CAD build for the part. Positions are in the model's coordinates, mm. Round coordinates to 2 decimals unless told otherwise and drop trailing zeros. Loops run counter-clockwise (first coordinate to the right, second up) from the corner with the lowest first, then second, coordinate; pieces in that order, holes last. Notation, with made-up numbers: (57.5, 55.5) -> (106.5, 55.5) arc R32 ccw to (106.5, 90.5) -> close; hole circle Ø11 at (-26.75, -40). An arc over 180 degrees is marked (long way). Answer as CSV lines item,"result".
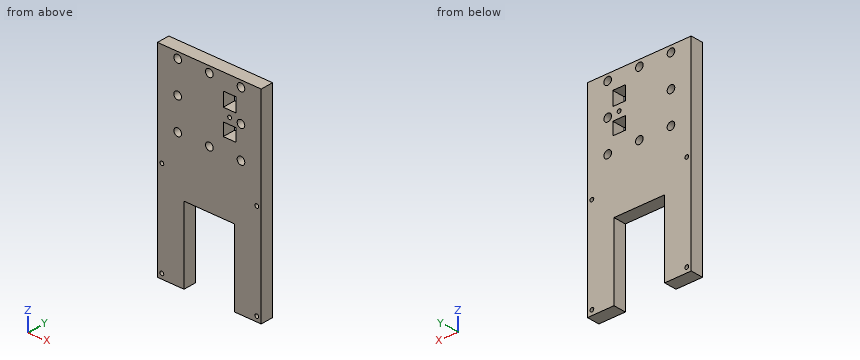
```python
from build123d import *

# Parameters (mm, degrees)
SKETCH1_R           = 3
SKETCH1_R_2         = 1.5
SKETCH1_W           = 10
SKETCH1_H           = 11
SKETCH1_H_2         = 10
BOSS_EXTRUDE1_DEPTH = 10


with BuildPart() as part:
    # Sketch1 → Boss-Extrude1 (new body)
    with BuildSketch(Plane(origin=(0, 0, 0), x_dir=(1, 0, 0), z_dir=(0, 1, 0))):
        Polygon((32.969203123, -64.744115369), (-49.030796877, -64.744115369), (-49.030796877, 95.255884631), (-28.030796877, 95.255884631), (-28.030796877, 35.255884631), (11.969203123, 35.255884631), (11.969203123, 95.255884631), (32.969203123, 95.255884631), align=None)
        with Locations(Location((-33.030796877, -59.744115369, 0), (0, 0, 270))):
            Circle(SKETCH1_R, mode=Mode.SUBTRACT)
        with Locations(Location((16.969203123, -59.744115369, 0), (0, 0, 270))):
            Circle(SKETCH1_R, mode=Mode.SUBTRACT)
        with Locations(Location((16.969203123, -9.744115369, 0), (0, 0, 270))):
            Circle(SKETCH1_R, mode=Mode.SUBTRACT)
        with Locations(Location((-33.030796877, -9.744115369, 0), (0, 0, 270))):
            Circle(SKETCH1_R, mode=Mode.SUBTRACT)
        with Locations(Location((-45.530796877, 91.255884631, 0), (0, 0, 270))):
            Circle(SKETCH1_R_2, mode=Mode.SUBTRACT)
        with Locations(Location((29.469203123, 91.255884631, 0), (0, 0, 270))):
            Circle(SKETCH1_R_2, mode=Mode.SUBTRACT)
        with Locations(Location((29.469203123, 16.255884631, 0), (0, 0, 270))):
            Circle(SKETCH1_R_2, mode=Mode.SUBTRACT)
        with Locations(Location((-45.530796877, 16.255884631, 0), (0, 0, 270))):
            Circle(SKETCH1_R_2, mode=Mode.SUBTRACT)
        with Locations(Location((-8.030796877, -9.744115369, 0), (0, 0, 270))):
            Circle(SKETCH1_R, mode=Mode.SUBTRACT)
        with Locations(Location((-33.030796877, -34.744115369, 0), (0, 0, 270))):
            Circle(SKETCH1_R, mode=Mode.SUBTRACT)
        with Locations(Location((16.969203123, -34.744115369, 0), (0, 0, 270))):
            Circle(SKETCH1_R, mode=Mode.SUBTRACT)
        with Locations(Location((-8.030796877, -59.744115369, 0), (0, 0, 270))):
            Circle(SKETCH1_R, mode=Mode.SUBTRACT)
        with Locations(Location((7.969203123, -35.744115369, 0), (0, 0, 270))):
            Circle(SKETCH1_R_2, mode=Mode.SUBTRACT)
        with Locations((7.969203123, -46.244115369)):
            Rectangle(SKETCH1_W, SKETCH1_H, mode=Mode.SUBTRACT)
        with Locations((7.969203123, -25.744115369)):
            Rectangle(SKETCH1_W, SKETCH1_H_2, mode=Mode.SUBTRACT)
    extrude(amount=BOSS_EXTRUDE1_DEPTH)


solid = part.part
```
Q1. Drop flat-ended pins along their axis: pin 1 Ø2.5 at (x, z) = (29.47, -16.26) entering from -Y; pin 2 Ø5 at (x, y) = (6.5, 3.5) entering from -Z. Give the stop position or say it passes through.
Results:
pin 1,"through"
pin 2,"z = -35.26"
Q2. Slice it at A-A, the plane z = -76. Give the cut face in (x, y), and give its area (3 significant figures).
Results:
outline,"(-49.03, 0) -> (-28.03, 0) -> (-28.03, 10) -> (-49.03, 10) -> close; (11.97, 0) -> (32.97, 0) -> (32.97, 10) -> (11.97, 10) -> close"
area,"420 mm2"
Q3. Probe L1, parallel to Z at x = 17, y = 1; L2, parallel to Z at x = -32.5, y = 4.75; L3, parallel to X at y = 6.5, z = 30.5. List the from-to ranges inside material, lowest first. Write a range as [from, to].
Results:
L1,"[-95.26, 6.74], [12.74, 31.74], [37.74, 56.74], [62.74, 64.74]"
L2,"[-95.26, 6.79], [12.7, 31.79], [37.7, 56.79], [62.7, 64.74]"
L3,"[-49.03, 2.97], [12.97, 32.97]"
Q4. Slice it at C-C, the plane x = -19.5. Give the cut face in (y, z).
Results:
outline,"(0, -35.26) -> (10, -35.26) -> (10, 64.74) -> (0, 64.74) -> close"
Q5. Slice it at B-B, the plane y = 3.75. Count the separate pieces of the cut face and the enclosed holes in it, and give its area (3 significant figures).
Results:
separate pieces,"1"
enclosed holes,"15"
area,"10,200 mm2"
